```python
from build123d import *

# Parameters (mm, degrees)
BOSS_EXTRUDE1_DEPTH      = 2.5
BOSS_EXTRUDE2_DEPTH      = 8.5
BOSS_EXTRUDE2_DEPTH_BACK = 3.25
SKETCH2_W                = 0.75
SKETCH2_H                = 0.75
CHAMFER1_SIZE            = 0.3


with BuildPart() as part:
    # Sketch1 → Boss-Extrude1 (new body)
    with BuildSketch(Plane(origin=(0, 0, 0), x_dir=(-1, 0, 0), z_dir=(0, 1, 0))):
        with BuildLine():
            Line((-17.25, 1.27), (2, 1.27))
            ThreePointArc((2, 1.27), (2.353553391, 1.123553391), (2.5, 0.77))
            Line((2.5, 0.77), (2.5, -0.77))
            ThreePointArc((2.5, -0.77), (2.353553391, -1.123553391), (2, -1.27))
            Line((2, -1.27), (-17.25, -1.27))
            ThreePointArc((-17.25, -1.27), (-17.603553391, -1.123553391), (-17.75, -0.77))
            Line((-17.75, -0.77), (-17.75, 0.77))
            ThreePointArc((-17.75, 0.77), (-17.603553391, 1.123553391), (-17.25, 1.27))
        make_face()
    extrude(amount=BOSS_EXTRUDE1_DEPTH)

    # Sketch2 → Boss-Extrude2 (add, two sides: drawn at the far end of the back side and taken through both)
    with BuildSketch(Plane(origin=(0, 0, 0), x_dir=(-1, 0, 0), z_dir=(0, 1, 0)).offset(-BOSS_EXTRUDE2_DEPTH_BACK)):
        with Locations((1.27, 0)):
            Rectangle(SKETCH2_W, SKETCH2_H)
        with Locations((-1.27, 0)):
            Rectangle(SKETCH2_W, SKETCH2_H)
        with Locations((-3.81, 0)):
            Rectangle(SKETCH2_W, SKETCH2_H)
        with Locations((-6.35, 0)):
            Rectangle(SKETCH2_W, SKETCH2_H)
        with Locations((-8.89, 0)):
            Rectangle(SKETCH2_W, SKETCH2_H)
        with Locations((-11.43, 0)):
            Rectangle(SKETCH2_W, SKETCH2_H)
        with Locations((-13.97, 0)):
            Rectangle(SKETCH2_W, SKETCH2_H)
        with Locations((-16.51, 0)):
            Rectangle(SKETCH2_W, SKETCH2_H)
    extrude(amount=BOSS_EXTRUDE2_DEPTH + BOSS_EXTRUDE2_DEPTH_BACK)

    # Chamfer1
    chamfer1_edges = [part.edges().sort_by_distance(p)[0] for p in [
        (9.265, -3.25, 0),
        (8.89, -3.25, 0.375),
        (8.515, -3.25, 0),
        (8.89, -3.25, -0.375),
        (9.265, 8.5, 0),
        (8.89, 8.5, -0.375),
        (8.515, 8.5, 0),
        (8.89, 8.5, 0.375),
        (11.055, -3.25, 0),
        (11.43, -3.25, -0.375),
        (11.805, -3.25, 0),
        (11.43, -3.25, 0.375),
        (11.055, 8.5, 0),
        (11.43, 8.5, 0.375),
        (11.805, 8.5, 0),
        (11.43, 8.5, -0.375),
        (14.345, -3.25, 0),
        (13.97, -3.25, 0.375),
        (13.595, -3.25, 0),
        (13.97, -3.25, -0.375),
        (14.345, 8.5, 0),
        (13.97, 8.5, -0.375),
        (13.595, 8.5, 0),
        (13.97, 8.5, 0.375),
        (16.135, -3.25, 0),
        (16.51, -3.25, -0.375),
        (16.885, -3.25, 0),
        (16.51, -3.25, 0.375),
        (16.135, 8.5, 0),
        (16.51, 8.5, 0.375),
        (16.885, 8.5, 0),
        (16.51, 8.5, -0.375),
        (-0.895, -3.25, 0),
        (-1.27, -3.25, 0.375),
        (-1.645, -3.25, 0),
        (-1.27, -3.25, -0.375),
        (-0.895, 8.5, 0),
        (-1.27, 8.5, -0.375),
        (-1.645, 8.5, 0),
        (-1.27, 8.5, 0.375),
        (0.895, -3.25, 0),
        (1.27, -3.25, -0.375),
        (1.645, -3.25, 0),
        (1.27, -3.25, 0.375),
        (0.895, 8.5, 0),
        (1.27, 8.5, 0.375),
        (1.645, 8.5, 0),
        (1.27, 8.5, -0.375),
        (4.185, -3.25, 0),
        (3.81, -3.25, 0.375),
        (3.435, -3.25, 0),
        (3.81, -3.25, -0.375),
        (4.185, 8.5, 0),
        (3.81, 8.5, -0.375),
        (3.435, 8.5, 0),
        (3.81, 8.5, 0.375),
        (5.975, -3.25, 0),
        (6.35, -3.25, -0.375),
        (6.725, -3.25, 0),
        (6.35, -3.25, 0.375),
        (5.975, 8.5, 0),
        (6.35, 8.5, 0.375),
        (6.725, 8.5, 0),
        (6.35, 8.5, -0.375),
    ]]
    chamfer(chamfer1_edges, length=CHAMFER1_SIZE)


solid = part.part
```
Design review of the part built by this model. Coordinates are the model's own, in mm. Coordinates: 2 decimals unless noted, no trailing zeros. Write each loop counter-clockwise with the first axis right and the second up, starting at its lowest first coordinate (ties: lowest second). Pieces come first, ordered by that corner, then holes.
1) To check wall thickness, follow L1, parallel to Y at x = 16.75, z = -0.5; L2, parallel to Z at x = 11.5, y = 5.5 (3 decimals); L3, parallel to X at y = 0.5, z = -1.1. State the ranges of each line that lie inside material, in increasing order.
2) Add section B-B (x = 12.25). Write out the cut boundary in (y, z).
3) Add section A-A (y = 4.75). State how many separate pieces and enclosed holes the cut face has, plus the area to 3 significant figures.
4) Mouldability with a two-part tool opening along X and no side actions: class faces 1 (the flat face through (7, 0, 0)), 2 (the flat face through (-2.5, 1, 0)), 3 (the flat face through (17.75, 1, 0)), 4 (the flat face through (7, 1, -1.27)) as +X half, -X half, draft (parallel to the pull), parting line (faces both ways), or undercut.
5) Insertion check: pin 1 (1 mm diameter, centred on x = 13.5, y = 4, fed in from -Z) (3 decimals); pin 2 (0.8 mm diameter, centred on y = 4.5, z = 0, fed in from +X) (3 decimals); pin 3 (0.6 mm diameter, centred on y = -1, z = 0, fed in from -X) (3 decimals). Each pin has a flat end and moves straight along its axis. Give the tip position at first contact, or say it passes through.
6) Add section C-C (z = 1). Write out the cut boundary in (x, y), plus the area to 3 significant figures.
Check result:
1. L1: y = 0 to 2.5
1. L2: z = -0.375 to 0.375
1. L3: x = -2.38 to 17.63
2. outline: (0, -1.27) - (2.5, -1.27) - (2.5, 1.27) - (0, 1.27) - close
3. separate pieces: 8
3. enclosed holes: 0
3. area: 4.50 mm2
4. face 1: undercut
4. face 2: -X half
4. face 3: +X half
4. face 4: draft
5. pin 1: stops at z = -0.375
5. pin 2: stops at x = 16.885
5. pin 3: stops at x = -1.645
6. outline: (-2.44, 0) - (17.69, 0) - (17.69, 2.5) - (-2.44, 2.5) - close
6. area: 50.3 mm2
